Here's how the part is built. I have some questions about the finished solid (model axes, mm). A direction names the side the tool comes from. Coordinates: 2 decimals unless noted, no trailing zeros. Loops run counter-clockwise (first coordinate to the right, second up) from the corner with the lowest first, then second, coordinate; pieces in that order, holes last. Notation, with made-up numbers: (-15.5, -37) -> (40.5, -37) arc R10 ccw to (40.5, -23) -> close; hole circle Ø6 at (75, 83.25). An arc over 180 degrees is marked (long way). Answer as a JSON object with one key per item and string values. Group by question number.
Q1. I want a section at B-B on z = -644. Write out the boundary of the cut face in (x, y), then the cut area to 3 significant figures.
Q2. I want a section at A-A on y = 7.25. Write out the boundary of the cut face in (x, z).
Q3. I need wall thicknesses on line 1 (X direction, y = 16.5, z = -664.5); line 2 (Z direction, x = -161.5, y = 5.5); line 3 (Z direction, x = -185, y = 9.75). Which ranges of each line are inside material? Lowest first, please.
Q4. On a 3-axis mill with a long thin cutter (end or side, diameter ignored), from which of +Z, -Z, +X, -X, +Y, -Y can I reach the whole of each face in a straight line? I mean faces 1 (the cylindrical face through (-159.632, 19.145, -351.59)), 2 (the cylindrical face through (-159.6, 0.9, -351.62)), 3 (the flat face through (-190.521, 10, -573)). Say none if no direction works.
Q5. Thinking about a two-plate mould opening in Z: for faces 4 (the flat face through (-132.84, 9.86, -311.73)), 5 (the cylindrical face through (-166.46, 19.1, -818.32)), 6 (the cylindrical face through (-151.51, 0.9, -807.41)), which applies, released by +Z, released by -Z, zero draft, split by the parting line, or undercut?
Q6. I'm going to push flat-ended pins straight in: pin 1 (5 mm diameter, centred on y = 6.5, z = -423, fed in from +X); pin 2 (6 mm diameter, centred on x = -143.5, y = 9, fed in from +Z); pin 3 (1 mm diameter, centred on x = -144, y = 15, fed in from -Z); pin 4 (5 mm diameter, centred on x = -191, z = -536.5, fed in from +Y). Where does each tip first touch, or does it pass through?
Autodesk Inventor part; units mm, degrees
ref_plane "YZ Plane" through (0, 0, 0) normal (1, 0, 0) x (0, 1, 0)
ref_plane "XZ Plane" through (0, 0, 0) normal (0, 1, 0) x (-1, 0, 0)
ref_plane "XY Plane" through (0, 0, 0) normal (0, 0, 1) x (1, 0, 0)
sketch "Sketch1" plane through (0, 0, 0) normal (0, 1, 0) x (-1, 0, 0)
  line L0 (909.7546, -1043.3394) -> (909.7546, -1834.2484) construction
  line L1 (909.7546, -1834.2484) -> (468.795, -1834.2484) construction
  line L2 (468.795, -1834.2484) -> (468.795, -1043.3394) construction
  line L3 (468.795, -1043.3394) -> (909.7546, -1043.3394) construction
  line L4 (1047.8435, -175.8693) -> (1047.8435, -771.5628) construction
  line L5 (1047.8435, -771.5628) -> (636.4111, -771.5628) construction
  line L6 (636.4111, -771.5628) -> (636.4111, -175.8693) construction
  line L7 (636.4111, -175.8693) -> (1047.8435, -175.8693) construction
  line L8 (-89.4601, -69.3306) -> (230.5399, -69.3306) construction
  line L9 (210.5212, -775.4703) -> (125.6684, -860.3231)
  line L10 (210.5212, -775.4703) -> (330.5212, -775.4703) construction
  line L11 (125.6684, -860.3231) -> (111.5263, -846.181)
  line L12 (210.5212, -775.4703) -> (210.5212, -375.4703)
  line L13 (210.5212, -775.4703) -> (610.5212, -775.4703) construction
  line L14 (210.5212, -375.4703) -> (139.8105, -304.7596)
  line L15 (139.8105, -304.7596) -> (125.6684, -318.9018)
  line L16 (125.6684, -318.9018) -> (182.2369, -375.4703)
  line L17 (190.5212, -767.186) -> (111.5263, -846.181)
  line L18 (190.5212, -383.7546) -> (182.2369, -375.4703)
  line L19 (190.5212, -383.7546) -> (190.5212, -767.186)
  dimension "d55" = 135
  dimension "d56" = 20
  dimension "d60" = 90
  dimension "d61" = 100
  dimension "d62" = 20
  dimension "d63" = 90
  dimension "d64" = 80
extrude "Extrusion2" add sketch "Sketch1" along normal blind 20
fillet "Fillet1" radius 3 14 edges at (-175.1659, 20, -340.115) (-175.1659, 0, -340.115) (-210.5212, 10, -375.4703) (-210.5212, 20, -575.4703) (-210.5212, 0, -575.4703) (-190.5212, 20, -575.4703) (-153.9527, 20, -347.186) (-151.0237, 20, -806.6835) (-151.0237, 0, -806.6835) (-210.5212, 10, -775.4703) (-168.0948, 0, -817.8967) (-168.0948, 20, -817.8967) (-190.5212, 0, -575.4703) (-153.9527, 0, -347.186)
properties part number "Suspension"
Result set:
{
 "1": {"outline": "(-210.52, 3) arc R3 ccw to (-207.52, 0) -> (-193.52, 0) arc R3 ccw to (-190.52, 3) -> (-190.52, 17) arc R3 ccw to (-193.52, 20) -> (-207.52, 20) arc R3 ccw to (-210.52, 17) -> close", "area": "392 mm²"},
 "2": {"outline": "(-210.52, -774.23) arc R3 ccw to (-209.64, -776.35) -> (-125.67, -860.32) -> (-111.53, -846.18) -> (-190.52, -767.19) -> (-190.52, -383.75) -> (-125.67, -318.9) -> (-139.81, -304.76) -> (-209.64, -374.59) arc R3 ccw to (-210.52, -376.71) -> close"},
 "3": {"line 1": "x = -210.52 to -190.52", "line 2": "z = -824.49 to -796.21, -354.73 to -326.45", "line 3": "z = -800.99 to -772.71, -378.23 to -349.95"},
 "4": {"face 1": "+X, +Y", "face 2": "+X, -Y", "face 3": "+X, +Y, -Y"},
 "5": {"face 4": "released by +Z", "face 5": "released by -Z", "face 6": "undercut"},
 "6": {"pin 1": "stops at x = -190.52", "pin 2": "stops at z = -305.45", "pin 3": "stops at z = -842.49", "pin 4": "stops at y = 20"}
}
